from build123d import *

# Parameters (mm, degrees)
BOSS_EXTRUDE1_DEPTH = 5
SKETCH3_W           = 2.6
SKETCH3_H           = 2.6
BOSS_EXTRUDE2_DEPTH = 5
SKETCH4_W           = 2.6
SKETCH4_H           = 2.6
BOSS_EXTRUDE3_DEPTH = 5
FILLET1_R           = 0.5


with BuildPart() as part:
    # Sketch2 → Boss-Extrude1 (new body)
    with BuildSketch(Plane.XY):
        with BuildLine():
            Line((1.75, -16.137999311), (-4, -16.137999311))
            Line((-4, -16.137999311), (-4, -17.137999311))
            Line((-4, -17.137999311), (4, -17.137999311))
            Line((4, -17.137999311), (4, -16.137999311))
            Line((4, -16.137999311), (3.164213562, -16.137999311))
            ThreePointArc((3.164213562, -16.137999311), (3.871320344, -13.637999311), (1.75, -12.137999311))
            Line((1.75, -12.137999311), (-2.5, -12.137999311))
            ThreePointArc((-2.5, -12.137999311), (-4.25, -10.387999311), (-2.5, -8.637999311))
            Line((-2.5, -8.637999311), (1.75, -8.637999311))
            ThreePointArc((1.75, -8.637999311), (4, -6.387999311), (1.75, -4.137999311))
            Line((1.75, -4.137999311), (-2.5, -4.137999311))
            ThreePointArc((-2.5, -4.137999311), (-4.25, -2.387999311), (-2.5, -0.637999311))
            Line((-2.5, -0.637999311), (1.75, -0.637999311))
            ThreePointArc((1.75, -0.637999311), (4, 1.612000689), (1.75, 3.862000689))
            Line((1.75, 3.862000689), (-2.5, 3.862000689))
            ThreePointArc((-2.5, 3.862000689), (-4.25, 5.612000689), (-2.5, 7.362000689))
            Line((-2.5, 7.362000689), (4, 7.362000689))
            Line((4, 7.362000689), (4, 8.362000689))
            Line((4, 8.362000689), (-4, 8.362000689))
            Line((-4, 8.362000689), (-4, 7.362000689))
            Line((-4, 7.362000689), (-3.914213562, 7.362000689))
            ThreePointArc((-3.914213562, 7.362000689), (-4.621320344, 4.862000689), (-2.5, 3.362000689))
            Line((-2.5, 3.362000689), (1.75, 3.362000689))
            ThreePointArc((1.75, 3.362000689), (3.5, 1.612000689), (1.75, -0.137999311))
            Line((1.75, -0.137999311), (-2.5, -0.137999311))
            ThreePointArc((-2.5, -0.137999311), (-4.75, -2.387999311), (-2.5, -4.637999311))
            Line((-2.5, -4.637999311), (1.75, -4.637999311))
            ThreePointArc((1.75, -4.637999311), (3.5, -6.387999311), (1.75, -8.137999311))
            Line((1.75, -8.137999311), (-2.5, -8.137999311))
            ThreePointArc((-2.5, -8.137999311), (-4.75, -10.387999311), (-2.5, -12.637999311))
            Line((-2.5, -12.637999311), (1.75, -12.637999311))
            ThreePointArc((1.75, -12.637999311), (3.5, -14.387999311), (1.75, -16.137999311))
        make_face()
    extrude(amount=BOSS_EXTRUDE1_DEPTH)

    # Sketch3 → Boss-Extrude2 (add)
    with BuildSketch(Plane(origin=(0, 8.362000689, 0), x_dir=(1, 0, 0), z_dir=(0, 1, 0))):
        with Locations((0, -2.5)):
            Rectangle(SKETCH3_W, SKETCH3_H)
    extrude(amount=BOSS_EXTRUDE2_DEPTH)

    # Sketch4 → Boss-Extrude3 (add)
    with BuildSketch(Plane.XZ.offset(17.137999311)):
        with Locations((0, 2.5)):
            Rectangle(SKETCH4_W, SKETCH4_H)
    extrude(amount=BOSS_EXTRUDE3_DEPTH)

    # Fillet1
    fillet1_edges = [part.edges().sort_by_distance(p)[0] for p in [
        (1.3, 10.862000689, 3.8),
        (1.3, 10.862000689, 1.2),
        (-1.3, 10.862000689, 1.2),
        (-1.3, 10.862000689, 3.8),
        (1.3, 13.362000689, 2.5),
        (0, 13.362000689, 1.2),
        (-1.3, 13.362000689, 2.5),
        (0, 13.362000689, 3.8),
        (-1.3, -19.637999311, 3.8),
        (-1.3, -19.637999311, 1.2),
        (1.3, -19.637999311, 1.2),
        (1.3, -19.637999311, 3.8),
        (-1.3, -22.137999311, 2.5),
        (0, -22.137999311, 1.2),
        (1.3, -22.137999311, 2.5),
        (0, -22.137999311, 3.8),
        (-4, 8.362000689, 2.5),
        (4, 8.362000689, 2.5),
        (4, -17.137999311, 2.5),
        (-4, -17.137999311, 2.5),
    ]]
    fillet(fillet1_edges, radius=FILLET1_R)


solid = part.part
Build history of the part. All positions in model axes, mm. A direction names the side the tool comes from. Coordinates: 2 decimals unless noted, no trailing zeros. Order: outer loops, then holes, each group sorted by start corner. A loop starts at its lowest first (then second) coordinate and runs counter-clockwise, first axis right, second up. Notation, with made-up numbers: M 66.5,87.5 L 115.5,87.5 A19 cw 115.5,107.5 Z; hole C 62,78 d5. An arc over 180 degrees is marked long. One line per question, with ' | ' between items. Start each with the question number.
Q1. 3-axis set-ups, long thin cutter, end or side, ignore diameter. For faces 1 (the face through (0, -4.638, 2)), 2 (the face through (1, 7.362, 2)), 3 (the face through (0, 11, 3.8)): which of +Z, -Z, +X, -X, +Y, -Y reach the whole face in a straight line?
Q2. Saw through at C-C (y = -14). List the corners of the cut face in (x, z).
Q3. Probe L1, parallel to X at y = -10.5, z = 4.7; L2, parallel to Y at x = 3.75, z = 3.85; L3, parallel to X at y = 9, z = 1.6. List the from-to ranges inside material, lowest first. Write a range as from..to.
Q4. Two-plate mould, pull along Y, no slides. Class faces 4 (the face through (0, -8.138, 2)), 5 (the face through (3.884, -13.675, 2.465)), 6 (the face through (0, 11, 1.2)): +Y half, -Y half, draft (parallel to the pull), parting line (faces both ways), or undercut.
Q5. Saw through at B-B (y = -9.5). List the corners of the cut face in (x, z), then the cut area to 3 significant figures.
Q6. Flat gauge pins, fed straight in: pin 1 Ø1.5 at (y, z) = (-2, 1.5) entering from +X; pin 2 Ø1 at (x, y) = (-2.5, -6) entering from +Z; pin 3 Ø0.8 at (x, y) = (0, 10.5) entering from +Z; pin 4 Ø0.8 at (y, z) = (-20, 2.5) entering from +X. Where does each tip first touch, or does it go through?
Q7. Saw through at A-A (x = 0). Count the separate pieces of the cut face and the enclosed holes in it, then the cut area to 3 significant figures.
Check values:
1) face 1: +Z, -Z, -X | face 2: +Z, -Z, +X | face 3: +Z, +X, -X, +Y
2) outline: M 3.46,0 L 3.97,0 L 3.97,5 L 3.46,5 Z
3) L1: x = -4.75..-4.25 | L2: y = -17.07..-16.14, -15.42..-13.36, -7.42..-5.36, 0.58..2.64, 7.36..8.3 | L3: x = -1.29..1.29
4) face 4: undercut | face 5: undercut | face 6: draft
5) outline: M -4.57,0 L -4.01,0 L -4.01,5 L -4.57,5 Z | area: 2.80 mm2
6) pin 1: stops at x = -3.83 | pin 2: passes through | pin 3: stops at z = 3.8 | pin 4: stops at x = 1.3
7) separate pieces: 7 | enclosed holes: 0 | area: 48.3 mm2
